Read the model definition and answer for the solid it produces. Units are mm, in the model's axes. A direction names the side the tool comes from. Round coordinates to 2 decimals unless told otherwise and drop trailing zeros. Write each loop counter-clockwise with the first axis right and the second up, starting at its lowest first coordinate (ties: lowest second). Pieces come first, ordered by that corner, then holes. Notation, with made-up numbers: (-16.75, -19.5) -> (25.25, -19.5) arc R20 ccw to (25.25, -10.5) -> close; hole circle Ø8 at (32, 34.5). An arc over 180 degrees is marked (long way). Return JSON: item names as keys, results as strings.
from build123d import *

# Parameters (mm, degrees)
BOSS_EXTRUDE1_DEPTH = 20.32
SKETCH2_W           = 120.284747719
SKETCH2_H           = 10.16
SKETCH2_W_2         = 118.872828106
SKETCH2_W_3         = 10.166490401
SKETCH2_H_2         = 89.916
SKETCH2_W_4         = 102.891608588
SKETCH2_W_5         = 94.453494603
SKETCH2_W_6         = 94.453494602
SKETCH2_W_7         = 3.175
SKETCH2_W_8         = 561.9496
CUT_EXTRUDE1_DEPTH  = 137.414
SKETCH3_W           = 337.058
SKETCH3_H           = 124.46
CUT_EXTRUDE2_DEPTH  = 137.414
SKETCH4_W           = 10.16
SKETCH4_H           = 63.685061479
SKETCH4_H_2         = 63.685061478
CUT_EXTRUDE3_DEPTH  = 20.32
SKETCH10_R          = 3.175
CUT_EXTRUDE5_DEPTH  = 20.32
SKETCH12_R          = 4.7625
CUT_EXTRUDE6_DEPTH  = 21.3200001
SKETCH14_R          = 3.175
CUT_EXTRUDE7_DEPTH  = 21.3200001
SKETCH15_R          = 4.7625
SKETCH15_R_2        = 3.175
CUT_EXTRUDE8_DEPTH  = 21.3200001
CUT_EXTRUDE9_DEPTH  = 21.3200001


with BuildPart() as part:
    # Sketch1 → Boss-Extrude1 (new body)
    with BuildSketch(Plane.XY):
        Polygon((94.041322477, 150.485716341), (-175.036761108, 150.485716341), (-142.097719316, 314.8709952), (61.102280684, 314.8709952), align=None)
        with BuildLine():
            Line((-606.997271248, -319.414283659), (526.001832617, -319.414283659))
            add(Edge.make_bspline(
                [(583.362059287, -282.457957765), (581.029219579, -287.649310181), (577.879080401, -292.734699958), (570.038270446, -301.965622016), (565.348976837, -306.100497209), (554.949172694, -312.800933616), (549.248266441, -315.360306939), (537.611112797, -318.678742027), (531.685117348, -319.440968422), (526.001832617, -319.414283659)],
                knots=[0, 0, 0, 0, 0.25, 0.25, 0.5, 0.5, 0.75, 0.75, 1, 1, 1, 1], degree=3))
            Line((583.362059287, -282.457957765), (777.91409763, 150.485716341))
            Line((777.91409763, 150.485716341), (-858.909536262, 150.485716341))
            Line((-858.909536262, 150.485716341), (-664.600308277, -281.91762311))
            add(Edge.make_bspline(
                [(-664.600308277, -281.91762311), (-662.275037436, -287.157802838), (-659.126015856, -292.295113907), (-651.27178065, -301.630322109), (-646.567903812, -305.817478055), (-636.124076479, -312.615880857), (-630.393770919, -315.220849348), (-618.687590773, -318.618481158), (-612.722057732, -319.414283659), (-606.997271248, -319.414283659)],
                knots=[0, 0, 0, 0, 0.25, 0.25, 0.5, 0.5, 0.75, 0.75, 1, 1, 1, 1], degree=3))
        make_face()
    extrude(amount=BOSS_EXTRUDE1_DEPTH)

    # Sketch2 → Cut-Extrude1 (cut)
    with BuildSketch(Plane(origin=(0, 0, 0), x_dir=(-1, 0, 0), z_dir=(0, 0, -1))):
        with Locations((-547.078117621, 145.405716341)):
            Rectangle(SKETCH2_W, SKETCH2_H)
        with Locations((-307.214581989, 145.405716341)):
            Rectangle(SKETCH2_W_2, SKETCH2_H)
        with Locations((-271.919035422, 5.451716341)):
            Rectangle(SKETCH2_W_3, SKETCH2_H_2)
        with Locations((-271.919035422, -174.380283659)):
            Rectangle(SKETCH2_W_3, SKETCH2_H_2)
        with Locations((352.914474055, -174.380283659)):
            Rectangle(SKETCH2_W_3, SKETCH2_H_2)
        with Locations((352.914474055, 5.451716341)):
            Rectangle(SKETCH2_W_3, SKETCH2_H_2)
        with Locations((380.219410862, 145.405716341)):
            Rectangle(SKETCH2_W_4, SKETCH2_H)
        with Locations((586.002628038, 145.405716341)):
            Rectangle(SKETCH2_W_4, SKETCH2_H)
        with Locations((-382.157322588, -314.334283659)):
            Rectangle(SKETCH2_W_5, SKETCH2_H)
        with Locations((463.152761219, -314.334283659)):
            Rectangle(SKETCH2_W_6, SKETCH2_H)
        with Locations((-278.589780623, -174.380283659)):
            Rectangle(SKETCH2_W_7, SKETCH2_H_2)
        with Locations((-265.248290222, -174.380283659)):
            Rectangle(SKETCH2_W_7, SKETCH2_H_2)
        with Locations((-278.589780623, 5.451716341)):
            Rectangle(SKETCH2_W_7, SKETCH2_H_2)
        with Locations((-265.248290222, 5.451716341)):
            Rectangle(SKETCH2_W_7, SKETCH2_H_2)
        with Locations((346.243728854, 5.451716341)):
            Rectangle(SKETCH2_W_7, SKETCH2_H_2)
        with Locations((359.585219255, 5.451716341)):
            Rectangle(SKETCH2_W_7, SKETCH2_H_2)
        with Locations((346.243728854, -174.380283659)):
            Rectangle(SKETCH2_W_7, SKETCH2_H_2)
        with Locations((359.585219255, -174.380283659)):
            Rectangle(SKETCH2_W_7, SKETCH2_H_2)
        with Locations((40.497719316, -314.334283659)):
            Rectangle(SKETCH2_W_8, SKETCH2_H)
    extrude(amount=-CUT_EXTRUDE1_DEPTH, mode=Mode.SUBTRACT)

    # Sketch3 → Cut-Extrude2 (cut)
    with BuildSketch(Plane.XY.offset(20.32)):
        with Locations((-40.497719316, -257.184283659)):
            Rectangle(SKETCH3_W, SKETCH3_H)
    extrude(amount=-CUT_EXTRUDE2_DEPTH, mode=Mode.SUBTRACT)

    # Sketch4 → Cut-Extrude3 (cut)
    with BuildSketch(Plane(origin=(0, 0, 0), x_dir=(-1, 0, 0), z_dir=(0, 0, -1))):
        Polygon((-160.162280684, -245.551796758), (-160.162280684, -309.254283659), (-128.031280684, -309.254283659), (-128.031280684, -194.954283659), (-150.002280684, -194.954283659), (-150.002280684, -245.551796758), align=None)
        Polygon((241.157719316, -309.254283659), (241.157719316, -245.551796758), (230.997719316, -245.551796758), (230.997719316, -194.954283659), (209.026719316, -194.954283659), (209.026719316, -309.254283659), align=None)
        with Locations((-155.082280684, -150.02420454)):
            Rectangle(SKETCH4_W, SKETCH4_H)
        with Locations((-155.082280684, -22.654081584)):
            Rectangle(SKETCH4_W, SKETCH4_H)
        with Locations((-155.082280684, 104.698615951)):
            Rectangle(SKETCH4_W, SKETCH4_H_2)
        with Locations((236.077719316, -150.02420454)):
            Rectangle(SKETCH4_W, SKETCH4_H)
        with Locations((236.077719316, -22.654081584)):
            Rectangle(SKETCH4_W, SKETCH4_H)
        with Locations((236.077719316, 104.698615951)):
            Rectangle(SKETCH4_W, SKETCH4_H_2)
    extrude(amount=-CUT_EXTRUDE3_DEPTH, mode=Mode.SUBTRACT)

    # Sketch10 → Cut-Extrude5 (cut)
    with BuildSketch(Plane.XY):
        with Locations((372.252552874, 80.840970313)):
            Circle(SKETCH10_R)
        with Locations((296.052552874, 80.840970313)):
            Circle(SKETCH10_R)
        with Locations((296.052552874, -8.059029687)):
            Circle(SKETCH10_R)
        with Locations((338.076100273, -8.059019539)):
            Circle(SKETCH10_R)
        with Locations((296.052552874, -96.959029687)):
            Circle(SKETCH10_R)
        with Locations((327.929280684, -242.858683659)):
            Circle(SKETCH10_R)
        with Locations((327.929280684, -268.258683659)):
            Circle(SKETCH10_R)
        with Locations((429.529280684, -268.258683659)):
            Circle(SKETCH10_R)
        with Locations((429.529280684, -242.858683659)):
            Circle(SKETCH10_R)
        with Locations((-510.524719316, -242.858683659)):
            Circle(SKETCH10_R)
        with Locations((-510.524719316, -268.258683659)):
            Circle(SKETCH10_R)
        with Locations((-408.924719316, -268.258683659)):
            Circle(SKETCH10_R)
        with Locations((-408.924719316, -242.858683659)):
            Circle(SKETCH10_R)
        with Locations((-377.047991505, -96.959029687)):
            Circle(SKETCH10_R)
        with Locations((-419.071538905, -8.059019539)):
            Circle(SKETCH10_R)
        with Locations((-377.047991505, -8.059029687)):
            Circle(SKETCH10_R)
        with Locations((-377.047991505, 80.840970313)):
            Circle(SKETCH10_R)
        with Locations((-453.247991505, 80.840970313)):
            Circle(SKETCH10_R)
    extrude(amount=CUT_EXTRUDE5_DEPTH, mode=Mode.SUBTRACT)

    # Sketch12 → Cut-Extrude6 (cut, through all)
    with BuildSketch(Plane(origin=(0, 0, 0), x_dir=(-1, 0, 0), z_dir=(0, 0, -1))):
        with Locations((-41.226780684, 125.085716341)):
            Circle(SKETCH12_R)
        with Locations((-41.226780684, 23.485716341)):
            Circle(SKETCH12_R)
        with Locations((-131.777780684, 23.485716341)):
            Circle(SKETCH12_R)
        with Locations((-131.777780684, 125.085716341)):
            Circle(SKETCH12_R)
        with Locations((212.773219316, 23.485716341)):
            Circle(SKETCH12_R)
        with Locations((212.773219316, 125.085716341)):
            Circle(SKETCH12_R)
        with Locations((122.222219316, 125.085716341)):
            Circle(SKETCH12_R)
        with Locations((122.222219316, 23.485716341)):
            Circle(SKETCH12_R)
    extrude(amount=-CUT_EXTRUDE6_DEPTH, mode=Mode.SUBTRACT)

    # Sketch14 → Cut-Extrude7 (cut, through all)
    with BuildSketch(Plane.XY.offset(20.32)):
        with Locations((435.255534848, 113.379343598)):
            Circle(SKETCH14_R)
        with Locations((485.903167936, 96.510716341)):
            Circle(SKETCH14_R)
        with Locations((485.903167936, 130.247970855)):
            Circle(SKETCH14_R)
    extrude(amount=-CUT_EXTRUDE7_DEPTH, mode=Mode.SUBTRACT)

    # Sketch15 → Cut-Extrude8 (cut, through all)
    with BuildSketch(Plane(origin=(0, 0, 0), x_dir=(-1, 0, 0), z_dir=(0, 0, -1))):
        with Locations((-54.752280684, -87.004283659)):
            Circle(SKETCH15_R)
        with Locations((135.747719316, -87.004283659)):
            Circle(SKETCH15_R)
        with Locations((40.497719316, -80.654283659)):
            Circle(SKETCH15_R_2)
    extrude(amount=-CUT_EXTRUDE8_DEPTH, mode=Mode.SUBTRACT)

    # Sketch16 → Cut-Extrude9 (cut, through all)
    with BuildSketch(Plane(origin=(0, 0, 0), x_dir=(-1, 0, 0), z_dir=(0, 0, -1))):
        Polygon((602.079238464, -249.356226254), (592.887014254, -245.028569373), (623.124185153, -180.802855087), (632.316409363, -185.130511968), align=None)
        Polygon((662.553580262, -120.904797683), (653.361356052, -116.577140802), (683.598526952, -52.351426516), (692.790751161, -56.679083397), align=None)
        Polygon((723.027922061, 7.546630889), (713.835697851, 11.87428777), (744.07286875, 76.100002056), (753.26509296, 71.772345174), align=None)
        Polygon((594.297271248, -319.414283659), (660.407848466, -275.75518023), (833.509536262, 109.454254463), (833.509536262, 150.485716341), (853.117470666, 153.088498724), (880.087987184, 153.088498724), (670.30731137, -269.21762311), (671.822506806, -327.097732355), (581.920341153, -337.589747111), align=None)
        Polygon((-752.51409763, 150.485716341), (-772.122032035, 153.088498724), (-799.092548552, 153.088498724), (-589.311872738, -269.21762311), (-590.827068174, -327.097732355), (-500.924902522, -337.589747111), (-513.301832617, -319.414283659), (-579.412409834, -275.75518023), (-752.51409763, 109.454254463), align=None)
        Polygon((-672.269654328, 71.772345174), (-663.077430118, 76.100002056), (-632.840259219, 11.87428777), (-642.032483429, 7.546630889), align=None)
        Polygon((-581.55814163, -120.904797683), (-611.795312529, -56.679083397), (-602.60308832, -52.351426516), (-572.365917421, -116.577140802), align=None)
        Polygon((-551.320970731, -185.130511968), (-542.128746521, -180.802855087), (-511.891575622, -245.028569373), (-521.083799832, -249.356226254), align=None)
    extrude(amount=-CUT_EXTRUDE9_DEPTH, mode=Mode.SUBTRACT)


solid = part.part
Item 1: Section C-C (x = -486.5) is taken. Give the vertices of the cut face in (y, z).
Worked answers:
{"outline": "(-309.25, 0) -> (150.49, 0) -> (150.49, 20.32) -> (-309.25, 20.32) -> close"}
Item 2: Straight lines are drawn through the part: L1, parallel to X at y = -137, z = 5.25; L2, parallel to X at y = 113, z = 11.75; L3, parallel to X at y = -74.5, z = 8.5. For each, find the intervals that lie inside material, in ascending order. Write a range as [from, to].
Worked answers:
{"L1": "x = [-722.76, -361.17], [-344.66, -241.16], [-231, 150], [160.16, 263.66], [280.18, 641.76]", "L2": "x = [-833.51, -241.16], [-231, 150], [160.16, 432.1], [438.41, 752.51]", "L3": "x = [-750.85, -684.4], [-673.17, 592.18], [603.41, 669.85]"}
Item 3: For a pull along Y with two mould halves and no side action, classify faces 1 (the flat face through (-668.27, -84.91, 10.02)), 2 (the flat face through (664.75, -85.85, 10.02)), 3 (the flat face through (-158.798, 231.528, 10.018)), 4 (the flat face through (656.94, 39.21, 10.02)) as released by +Y, released by -Y, zero draft, split by the parting line, or undercut.
Worked answers:
{"face 1": "undercut", "face 2": "released by -Y", "face 3": "released by +Y", "face 4": "undercut"}
Item 4: Flat-ended cylindrical pins translate along their axes: pin 1 (4 mm diameter, centred on y = 170, z = 14.5, fed in from -X); pin 2 (4 mm diameter, centred on x = -510.52, y = -242.86, fed in from -Z); pin 3 (5 mm diameter, centred on y = -314, z = 9.5, fed in from -X); pin 4 (1.5 mm diameter, centred on y = -17, z = 7, fed in from +X). Find the tip coordinate at first contact, or state that the pin passes through.
Worked answers:
{"pin 1": "stops at x = -171.53", "pin 2": "passes through", "pin 3": "stops at x = -606.28", "pin 4": "stops at x = 696.03"}
Item 5: A tool of negligible diameter and unlimited length cuts with its end or side. For faces 5 (the flat face through (596.465, -89.242, 10.018)), 6 (the flat face through (77.34, 233.83, 10.02)), from which of +Z, -Z, +X, -X, +Y, -Y can it reach the whole face along a straight path? Write none if from no direction.
Worked answers:
{"face 5": "+Z, -Z", "face 6": "+Z, -Z, +X, +Y"}
Item 6: Section B-B (z = 16.5) is taken. State how many separate pieces and enclosed holes the cut face has, then the cut area to 3 significant figures.
Worked answers:
{"separate pieces": "1", "enclosed holes": "48", "area": "627,000 mm2"}
Item 7: Section A-A (x = 14) is taken. Give the vertices of the cut face in (y, z).
Worked answers:
{"outline": "(-194.95, 0) -> (314.87, 0) -> (314.87, 20.32) -> (-194.95, 20.32) -> close"}
